Geometry check sheet. Reference: the model listing, model coordinates, mm. A direction names the side the tool comes from. Coordinates: 2 decimals unless noted, no trailing zeros. Write each loop counter-clockwise with the first axis right and the second up, starting at its lowest first coordinate (ties: lowest second). Pieces come first, ordered by that corner, then holes. Notation, with made-up numbers: (-13.5, 23.25) -> (14.5, 23.25) arc R18 ccw to (14.5, 30.25) -> close; hole circle Ø1 at (21, 49). An arc over 180 degrees is marked (long way). Answer as CSV lines item,"result".
```python
from build123d import *

# Parameters (mm, degrees)
SKETCH_1_W          = 300
SKETCH_1_H          = 165
EXTRUDE_1_DEPTH     = 10
SKETCH_2_W          = 40
SKETCH_2_H          = 40
EXTRUDE_2_DEPTH     = 20
EXTRUDE_3_DEPTH     = 50
SKETCH_5_R          = 8
CUT_EXTRUDE_1_DEPTH = 348.598906788


with BuildPart() as part:
    # 스케치1 → 보스-돌출1 (new body)
    with BuildSketch(Plane.XY):
        with Locations((150, 82.5)):
            Rectangle(SKETCH_1_W, SKETCH_1_H)
    extrude(amount=EXTRUDE_1_DEPTH)

    # 스케치2 → 보스-돌출2 (add)
    with BuildSketch(Plane.XY.offset(10)):
        with Locations((20, 82.5)):
            Rectangle(SKETCH_2_W, SKETCH_2_H)
        with Locations((280, 82.5)):
            Rectangle(SKETCH_2_W, SKETCH_2_H)
    extrude(amount=EXTRUDE_2_DEPTH)

    # 스케치4 → 보스-돌출3 (add)
    with BuildSketch(Plane.XY.offset(10)):
        Polygon((0, 165), (0, 102.5), (10, 102.5), (10, 155), (290, 155), (290, 102.5), (300, 102.5), (300, 165), align=None)
        Polygon((10, 62.5), (0, 62.5), (0, 0), (300, 0), (300, 62.5), (290, 62.5), (290, 10), (10, 10), align=None)
    extrude(amount=EXTRUDE_3_DEPTH)

    # 스케치5 → 컷-돌출1 (cut, through all)
    with BuildSketch(Plane(origin=(300, 0, 0), x_dir=(0, 0, -1), z_dir=(1, 0, 0))):
        with Locations((-30, 82.5)):
            Circle(SKETCH_5_R)
    extrude(amount=-CUT_EXTRUDE_1_DEPTH, mode=Mode.SUBTRACT)


solid = part.part
```
Item 1: Thickness scan on probe 1 along Y at (x, z) = (18.5, 34); probe 2 along X at (y, z) = (133, 13); probe 3 along X at (y, z) = (90, 24). Record the ranges inside material, lowest first.
Responses:
probe 1,"y = 0 to 10, 155 to 165"
probe 2,"x = 0 to 10, 290 to 300"
probe 3,"x = 0 to 40, 260 to 300"
Item 2: Cross-section at D-D, the plane y = 82.5. Record the cut outline in (x, z), plus the area to 3 significant figures.
Responses:
outline,"(0, 0) -> (300, 0) -> (300, 22) -> (260, 22) -> (260, 10) -> (40, 10) -> (40, 22) -> (0, 22) -> close"
area,"3,960 mm2"
Item 3: Release check for a two-part mould opening along Y. For faces 1 (the flat face through (260, 82, 20)), 2 (the flat face through (148, 0, 30)), 3 (the flat face through (149, 157, 60)) record: +Y half, -Y half, draft (parallel to the pull), parting line (faces both ways), or undercut.
Responses:
face 1,"undercut"
face 2,"-Y half"
face 3,"draft"
Item 4: Cross-section at C-C, the plane x = 237. Record the cut outline in (y, z).
Responses:
outline,"(0, 0) -> (165, 0) -> (165, 60) -> (155, 60) -> (155, 10) -> (10, 10) -> (10, 60) -> (0, 60) -> close"
Item 5: Cross-section at B-B, the plane z = 36. Record the cut outline in (x, y).
Responses:
outline,"(0, 0) -> (300, 0) -> (300, 62.5) -> (290, 62.5) -> (290, 10) -> (10, 10) -> (10, 62.5) -> (0, 62.5) -> close; (0, 102.5) -> (10, 102.5) -> (10, 155) -> (290, 155) -> (290, 102.5) -> (300, 102.5) -> (300, 165) -> (0, 165) -> close"
Item 6: Set-up check for faces 4 (the flat face through (5, 62.5, 45)), 5 (the flat face through (0, 84, 16)), 6 (the flat face through (290, 129, 35)): record each of +Z, -Z, +X, -X, +Y, -Y from which the full face is reachable in a straight line by a thin tool's end or side.
Responses:
face 4,"+Z, +X, -X"
face 5,"+Z, -Z, -X, +Y, -Y"
face 6,"+Z"
Item 7: Cross-section at A-A, the plane z = 14. Record the cut outline in (x, y), plus the area to 3 significant figures.
Responses:
outline,"(0, 0) -> (300, 0) -> (300, 165) -> (0, 165) -> close; hole (10, 10) -> (290, 10) -> (290, 62.5) -> (260, 62.5) -> (260, 102.5) -> (290, 102.5) -> (290, 155) -> (10, 155) -> (10, 102.5) -> (40, 102.5) -> (40, 62.5) -> (10, 62.5) -> close"
area,"11,300 mm2"
Item 8: Depth check by flat-ended pin: pin 1 Ø8 at (x, y) = (161, 31.5) entering from +Z; pin 2 Ø13 at (x, y) = (274, 94.5) entering from +Z. Enter the tip coordinate at first touch or a pass-through.
Responses:
pin 1,"stops at z = 10"
pin 2,"stops at z = 30"
